Verification items for the finished model (mm, model axes). A direction names the side the tool comes from. Give positions to 0.01 mm unless a question says otherwise; leave off trailing zeros. Order: outer loops, then holes, each group sorted by start corner. A loop starts at its lowest first (then second) coordinate and runs counter-clockwise, first axis right, second up. Notation, with made-up numbers: (67.5, 85) - (102.5, 85) arc R14 ccw to (102.5, 105) - close; hole circle Ø4 at (81, 62.5). An arc over 180 degrees is marked (long way). Answer as a JSON object with one key per item and string values. Group by question number.
(1) Section check A-A (x = 18.5). Record the boundary of the cut face in (y, z), then the cut area to 3 significant figures.
(2) Section check C-C (y = -9). Record the boundary of the cut face in (x, z).
(3) Section check B-B (z = 119). Record the boundary of the cut face in (x, y), then the cut area to 3 significant figures.
(4) Mould release check, pull along Z, two halves, no side actions. Record for faces 1 (the face through (31, 1, 0)), 2 (the face through (31, 1, 130)), 3 (the face through (28.773, 3, 113)), 4 (the face through (0, 3, 64)): +Z half, -Z half, draft (parallel to the pull), parting line (faces both ways), or undercut.
(5) Thickness scan on line 1 (X direction, y = 0.5, z = 116.5); line 2 (X direction, y = -33.5, z = 82.5); line 3 (Y direction, x = 35, z = 60). Record the ranges inside material, lowest first.
(6) Section check D-D (z = 39). Record the boundary of the cut face in (x, y).
(7) Access from +Z, -Z, +X, -X, +Y, -Y to the whole of each face (thin tool, end or side, straight path). Record for faces 5 (the face through (15.773, 3, 113)), 6 (the face through (40, -20, 64)), 7 (the face through (23, 5, 64)).
(8) Depth check by flat-ended pin: pin 1 Ø10 at (y, z) = (-24, 57.5) entering from -X; pin 2 Ø12 at (x, z) = (19, 48) entering from -Y. Enter the tip coordinate at first touch or a pass-through.
```python
from build123d import *

# Parameters (mm, degrees)
BOSS_EXTRUDE1_DEPTH = 130
CUT_EXTRUDE1_DEPTH  = 10


with BuildPart() as part:
    # Sketch2 → Boss-Extrude1 (new body)
    with BuildSketch(Plane.XY):
        Polygon((0, 0), (40, 0), (40, -40), (45, -40), (45, 5), (0, 5), align=None)
    extrude(amount=BOSS_EXTRUDE1_DEPTH)

    # Sketch3 → Cut-Extrude1 (cut)
    with BuildSketch(Plane(origin=(0, 5, 0), x_dir=(1, 0, 0), z_dir=(0, 1, 0))):
        with BuildLine():
            Line((28.773082799, -14), (28.773082799, -20))
            ThreePointArc((28.773082799, -20), (22.273082799, -26.5), (15.773082799, -20))
            Line((15.773082799, -20), (15.773082799, -14))
            ThreePointArc((15.773082799, -14), (22.273082799, -7.5), (28.773082799, -14))
        make_face()
        with BuildLine():
            Line((28.773082799, -116), (28.773082799, -110))
            ThreePointArc((28.773082799, -110), (22.273082799, -103.5), (15.773082799, -110))
            Line((15.773082799, -110), (15.773082799, -116))
            ThreePointArc((15.773082799, -116), (22.273082799, -122.5), (28.773082799, -116))
        make_face()
    extrude(amount=-CUT_EXTRUDE1_DEPTH, mode=Mode.SUBTRACT)


solid = part.part
```
Solutions:
{
 "1": {"outline": "(0, 0) - (5, 0) - (5, 8.71) - (0, 8.71) - close; (0, 25.29) - (5, 25.29) - (5, 104.71) - (0, 104.71) - close; (0, 121.29) - (5, 121.29) - (5, 130) - (0, 130) - close", "area": "484 mm2"},
 "2": {"outline": "(40, 0) - (45, 0) - (45, 130) - (40, 130) - close"},
 "3": {"outline": "(0, 0) - (16.51, 0) - (16.51, 5) - (0, 5) - close; (28.04, 0) - (40, 0) - (40, -40) - (45, -40) - (45, 5) - (28.04, 5) - close", "area": "367 mm2"},
 "4": {"face 1": "-Z half", "face 2": "+Z half", "face 3": "undercut", "face 4": "draft"},
 "5": {"line 1": "x = 0 to 15.79, 28.75 to 45", "line 2": "x = 40 to 45", "line 3": "y = 0 to 5"},
 "6": {"outline": "(0, 0) - (40, 0) - (40, -40) - (45, -40) - (45, 5) - (0, 5) - close"},
 "7": {"face 5": "+Y, -Y", "face 6": "+Z, -Z, -X, -Y", "face 7": "+Z, -Z, +X, -X, +Y"},
 "8": {"pin 1": "stops at x = 40", "pin 2": "stops at y = 0"}
}
